Autodesk Inventor part; units mm, degrees
ref_plane "YZ Plane" through (0, 0, 0) normal (1, 0, 0) x (0, 1, 0)
ref_plane "XZ Plane" through (0, 0, 0) normal (0, 1, 0) x (-1, 0, 0)
ref_plane "XY Plane" through (0, 0, 0) normal (0, 0, 1) x (1, 0, 0)
sketch "Sketch1" plane through (0, 0, 0) normal (0, 0, 1) x (1, 0, 0)
  line L0 (0, 0) -> (4, 0)
  line L1 (4, 0) -> (4, 24)
  line L2 (4, 24) -> (0, 24)
  line L3 (0, 24) -> (0, 0)
  dimension "d0" = 4
  dimension "d1" = 24
extrude "Extrusion1" add sketch "Sketch1" along normal blind 200
fillet "Fillet1" radius 5 4 edges at (2, 24, 200) (2, 0, 200) (2, 24, 0) (2, 0, 0)
sketch "Sketch2" plane through (4, 5, 0) normal (1, 0, 0) x (0, 0, -1)
  circle A0 centre (-50, 7) radius 4
  circle A1 centre (-150, 7) radius 4
  line L0 (-200, 0) -> (-200, 14)
  line L1 (0, 0) -> (0, 14)
  line L2 (-5, 19) -> (-195, 19)
  circle A2 centre (-175, 7) radius 4
  circle A3 centre (-25, 7) radius 4
  circle A4 centre (-115, 7) radius 4
  circle A5 centre (-85, 7) radius 4
  point P0 (0, -5)
  dimension "d5" = 8
  dimension "d6" = 8
  dimension "d9" = 50
  dimension "d10" = 50
  dimension "d11" = 12
  dimension "d12" = 12
  dimension "d13" = 8
  dimension "d14" = 8
  dimension "d15" = 8
  dimension "d16" = 8
  dimension "d17" = 25
  dimension "d18" = 25
  dimension "d19" = 85
  dimension "d20" = 85
extrude "Extrusion2" cut sketch "Sketch2" against normal up to surface (4 mm away)
sketch "Sketch3" plane through (4, 5, 0) normal (1, 0, 0) x (0, 0, -1)
  point P0 (0, -5)
properties part number "mocowanie zawieszenia"
The model under review builds one solid part; all positions refer to its coordinate system, in mm. Coordinates: 2 decimals unless noted, no trailing zeros. Order: outer loops, then holes, each group sorted by start corner. A loop starts at its lowest first (then second) coordinate and runs counter-clockwise, first axis right, second up. Notation, with made-up numbers: (20, 43) -> (79, 43) arc R23 ccw to (79, 74) -> close; hole circle Ø7 at (-8.75, -12.5). An arc over 180 degrees is marked (long way). Answer in a Markdown table with one row per item.
(1) Insertion check: pin 1 (2 mm diameter, centred on x = 3.5, y = 2.5, fed in from -Z). The pin has a flat end and moves straight along its axis. Give the tip position at first contact, or say it passes through.
Answers:
| item | result |
|---|---|
| pin 1 | z = 0.23 |
(2) Consider section B-B (z = 25). Write out the cut boundary in (x, y).
Answers:
| item | result |
|---|---|
| outline | (0, 0) -> (4, 0) -> (4, 8) -> (0, 8) -> close; (0, 16) -> (4, 16) -> (4, 24) -> (0, 24) -> close |
(3) Consider section A-A (y = 12). Write out the cut boundary in (x, z), plus the area to 3 significant figures.
Answers:
| item | result |
|---|---|
| outline | (0, 0) -> (4, 0) -> (4, 21) -> (0, 21) -> close; (0, 29) -> (4, 29) -> (4, 46) -> (0, 46) -> close; (0, 54) -> (4, 54) -> (4, 81) -> (0, 81) -> close; (0, 89) -> (4, 89) -> (4, 111) -> (0, 111) -> close; (0, 119) -> (4, 119) -> (4, 146) -> (0, 146) -> close; (0, 154) -> (4, 154) -> (4, 171) -> (0, 171) -> close; (0, 179) -> (4, 179) -> (4, 200) -> (0, 200) -> close |
| area | 608 mm² |
(4) Wall thickness on line 1 along Y through (x, z) = (1.25, 50); line 2 along Y through (x, z) = (2.7, 174); line 3 along Z through (x, y) = (1.3, 21): over which ranges is each line inside the solid? List them lowest first.
Answers:
| item | result |
|---|---|
| line 1 | 0 to 8, 16 to 24 |
| line 2 | 0 to 8.13, 15.87 to 24 |
| line 3 | 0.42 to 199.58 |
(5) The part is to be moulded in two halves that separate along Z. For faces 1 (the cylindrical face through (2, 23, 2)), 2 (the cylindrical face through (2.028, 13.201, 146.185)), 3 (the cylindrical face through (2, 2, 199)), say which applies: +Z half, -Z half, draft (parallel to the pull), parting line (faces both ways), or undercut.
Answers:
| item | result |
|---|---|
| face 1 | -Z half |
| face 2 | undercut |
| face 3 | +Z half |
(6) Consider section C-C (x = 0.6). Write out the cut boundary in (y, z).
Answers:
| item | result |
|---|---|
| outline | (0, 5) arc R5 ccw to (5, 0) -> (19, 0) arc R5 ccw to (24, 5) -> (24, 195) arc R5 ccw to (19, 200) -> (5, 200) arc R5 ccw to (0, 195) -> close; hole circle Ø8 at (12, 25); hole circle Ø8 at (12, 50); hole circle Ø8 at (12, 85); hole circle Ø8 at (12, 115); hole circle Ø8 at (12, 150); hole circle Ø8 at (12, 175) |
